Design review of the part built by this model. Coordinates are the model's own, in mm. Coordinates: 2 decimals unless noted, no trailing zeros. Loops run counter-clockwise (first coordinate to the right, second up) from the corner with the lowest first, then second, coordinate; pieces in that order, holes last. Notation, with made-up numbers: (-3.75, 17.25) -> (27.25, 17.25) arc R28 cw to (27.25, 47.25) -> close; hole circle Ø5 at (65.5, -25.75). An arc over 180 degrees is marked (long way). Use CSV: the item, a comma, the result in double quotes.
```python
from build123d import *

# Parameters (mm, degrees)
F0_R     = 2.5
F2_DEPTH = 170


with BuildPart() as f2:
    # F0 (on Front) → F2 (new body)
    with BuildSketch(Plane.XZ):
        with BuildLine():
            Line((6.5, 0), (2, 0))
            ThreePointArc((2, 0), (0.5857864376, -0.5857864376), (0, -2))
            Line((0, -2), (0, -6.4857100192))
            Line((0, -6.4857100192), (0.4948230833, -6.489995392))
            Line((0.4948230833, -6.489995392), (0.4948230833, -7))
            Line((0.4948230833, -7), (2, -7))
            Line((2, -7), (2, -3.0833937817))
            Line((2, -3.0833937817), (6.2, -7.2637052917))
            Line((6.2, -7.2637052917), (6.2, -12.7393398282))
            Line((6.2, -12.7393398282), (2, -16.9393398282))
            Line((2, -16.9393398282), (2, -13))
            Line((2, -13), (0.5, -13))
            Line((0.5, -13), (0.5, -13.5))
            Line((0.5, -13.5), (0, -13.5))
            Line((0, -13.5), (0, -18))
            ThreePointArc((0, -18), (0.5857864376, -19.4142135624), (2, -20))
            Line((2, -20), (6.5, -20))
            Line((6.5, -20), (6.5, -19.5))
            Line((6.5, -19.5), (7, -19.5))
            Line((7, -19.5), (7, -18))
            Line((7, -18), (3.0606601718, -18))
            Line((3.0606601718, -18), (7.2606601718, -13.8))
            Line((7.2606601718, -13.8), (12.7393398282, -13.8))
            Line((12.7393398282, -13.8), (16.9393398282, -18))
            Line((16.9393398282, -18), (13.015800612, -18))
            Line((13.015800612, -18), (13.015800612, -19.5))
            Line((13.015800612, -19.5), (13.5, -19.5))
            Line((13.5, -19.5), (13.5, -20))
            Line((13.5, -20), (18, -20))
            ThreePointArc((18, -20), (19.4142135624, -19.4142135624), (20, -18))
            Line((20, -18), (20, -13.4626608249))
            Line((20, -13.4626608249), (19.5363645284, -13.4624647606))
            Line((19.5363645284, -13.4624647606), (19.532302618, -12.9822008219))
            Line((19.532302618, -12.9822008219), (18, -12.9822008219))
            Line((18, -12.9822008219), (17.9998106987, -16.9393398192))
            Line((17.9998106987, -16.9393398192), (13.8264202785, -12.765949399))
            Line((13.8264202785, -12.765949399), (13.8264202785, -7.246708479))
            Line((13.8264202785, -7.246708479), (17.9998106987, -3.0606601627))
            Line((17.9998106987, -3.0606601627), (17.9998106987, -6.9999999909))
            Line((17.9998106987, -6.9999999909), (19.4998106987, -6.9999999909))
            Line((19.4998106987, -6.9999999909), (19.4998106987, -6.4999999909))
            Line((19.4998106987, -6.4999999909), (20, -6.4999999909))
            Line((20, -6.4999999909), (20, -2))
            ThreePointArc((20, -2), (19.4142135624, -0.5857864376), (18, 0))
            Line((18, 0), (13.4962801728, 0.0202495232))
            Line((13.4962801728, 0.0202495232), (13.5, -0.5))
            Line((13.5, -0.5), (13.015800612, -0.5))
            Line((13.015800612, -0.5), (13.015800612, -2))
            Line((13.015800612, -2), (16.9393398282, -2))
            Line((16.9393398282, -2), (12.7393121854, -6.2000276428))
            Line((12.7393121854, -6.2000276428), (7.2606601718, -6.2))
            Line((7.2606601718, -6.2), (3.0606601718, -2))
            Line((3.0606601718, -2), (7, -2))
            Line((7, -2), (7, -0.5))
            Line((7, -0.5), (6.5, -0.5))
            Line((6.5, -0.5), (6.5, 0))
        make_face()
        with Locations((10, -10)):
            Circle(F0_R, mode=Mode.SUBTRACT)
    extrude(amount=F2_DEPTH)


solid = f2.part
```
Item 1: Add section A-A (z = -10). Give the boundary of the cut face in (x, y), then the cut area to 3 significant figures.
Checked values:
outline,"(6.2, -170) -> (7.5, -170) -> (7.5, 0) -> (6.2, 0) -> close; (12.5, -170) -> (13.83, -170) -> (13.83, 0) -> (12.5, 0) -> close"
area,"446 mm^2"
Item 2: Draft analysis for pull direction Z (two halves, no side actions). For faces 1 (the face through (5.13, -83.81, -15.93)), 2 (the face through (5, -84, -18)), 3 (the face through (20, -84, -16)), 4 (the face through (16, -84, -20)), state which applies: pulls with the +Z half, pulls with the -Z half, needs draft (parallel to the pull), parting line crosses it, or undercut.
Checked values:
face 1,"undercut"
face 2,"undercut"
face 3,"needs draft"
face 4,"pulls with the -Z half"
Item 3: To check wall thickness, follow line 1 along X through (y, z) = (-48, -6.25); line 2 along X through (y, z) = (-10, -3.25); line 3 along Z through (x, y) = (10, -100). State the ranges of each line that lie inside material, in increasing order.
Checked values:
line 1,"0 to 2, 5.18 to 14.82, 18 to 20"
line 2,"0 to 2, 2.17 to 4.31, 15.69 to 17.81, 18 to 20"
line 3,"-13.8 to -12.5, -7.5 to -6.2"
Item 4: Clearance check with flat-ended pins moving along their axes: pin 1 (6 mm diameter, centred on x = 14.5, z = -9.5, fed in from +Y); pin 2 (6 mm diameter, centred on x = 17, y = -73.5, fed in from +Z); pin 3 (1 mm diameter, centred on x = 10.5, z = -14.5, fed in from -Y); pin 4 (4.5 mm diameter, centred on y = -45, z = -9, fed in from -X). State where each tip first meets the part, or that it passes through.
Checked values:
pin 1,"y = 0"
pin 2,"z = 0.02"
pin 3,"through"
pin 4,"x = 0.49"
Item 5: Add section B-B (x = 4.75). Give the boundary of the cut face in (y, z), then the cut area to 3 significant figures.
Checked values:
outline,"(-170, -20) -> (0, -20) -> (0, -18) -> (-170, -18) -> close; (-170, -16.31) -> (0, -16.31) -> (0, -14.19) -> (-170, -14.19) -> close; (-170, -5.82) -> (0, -5.82) -> (0, -3.69) -> (-170, -3.69) -> close; (-170, -2) -> (0, -2) -> (0, 0) -> (-170, 0) -> close"
area,"1,400 mm^2"
